```python
from build123d import *

# Parameters (mm, degrees)
EXTRUDE_1_DEPTH           = 12.5
CUT_EXTRUDE_1_DEPTH       = 20.532024985
CUT_EXTRUDE_1_DEPTH_BACK  = 20.532024985
SKETCH_2_R                = 2
CUT_EXTRUDE_2_DEPTH       = 20.532024985
CUT_EXTRUDE_2_DEPTH_BACK  = 20.532024985
CUT_EXTRUDE_START         = 12.5
SKETCH_5_W                = 16
SKETCH_5_H                = 5
CUT_EXTRUDE_4_DEPTH       = 5.5
CUT_EXTRUDE_5_DEPTH       = 2.5
CUT_EXTRUDE_5_DEPTH_BACK  = 2.5
EXTRUDE_START             = 12.5
EXTRUDE_5_DEPTH           = 1.5
SKETCH_8_R                = 1
CUT_EXTRUDE_6_DEPTH       = 1.5
CUT_EXTRUDE_START_2       = 14
CUT_EXTRUDE_7_DEPTH       = 1.5
CUT_EXTRUDE_9_DEPTH       = 29.943911277
CUT_EXTRUDE_9_DEPTH_BACK  = 29.943911277
CUT_EXTRUDE_10_DEPTH      = 29.943911277
CUT_EXTRUDE_10_DEPTH_BACK = 29.943911277


with BuildPart() as part:
    # 草图1 → 凸台-拉伸1 (new body)
    with BuildSketch(Plane(origin=(0, 0, 0), x_dir=(1, 0, 0), z_dir=(0, 1, 0))):
        Polygon((13, 5.5), (8, 5.5), (8, -5.5), (13, -5.5), (13, -7.5), (-13, -7.5), (-13, -5.5), (-8, -5.5), (-8, 5.5), (-13, 5.5), (-13, 7.5), (13, 7.5), align=None)
    extrude(amount=EXTRUDE_1_DEPTH)

    # 草图2 → 切除-拉伸1 (cut, two sides: drawn at the far end of the back side and taken through both)
    with BuildSketch(Plane.XY.offset(-CUT_EXTRUDE_1_DEPTH_BACK)):
        with Locations((0, 3.5)):
            Circle(SKETCH_2_R)
    extrude(amount=CUT_EXTRUDE_1_DEPTH + CUT_EXTRUDE_1_DEPTH_BACK, mode=Mode.SUBTRACT)

    # 草图3 → 切除-拉伸2 (cut, two sides: drawn at the far end of the back side and taken through both)
    with BuildSketch(Plane.XY.offset(-CUT_EXTRUDE_2_DEPTH_BACK)):
        with BuildLine():
            Line((-10.5, 11), (-2, 11))
            ThreePointArc((-2, 11), (-1, 10), (-2, 9))
            Line((-2, 9), (-10.5, 9))
            ThreePointArc((-10.5, 9), (-11.5, 10), (-10.5, 11))
        make_face()
        with BuildLine():
            Line((2, 9), (10.5, 9))
            ThreePointArc((10.5, 9), (11.5, 10), (10.5, 11))
            Line((10.5, 11), (2, 11))
            ThreePointArc((2, 11), (1, 10), (2, 9))
        make_face()
    extrude(amount=CUT_EXTRUDE_2_DEPTH + CUT_EXTRUDE_2_DEPTH_BACK, mode=Mode.SUBTRACT)

    # 草图5 → 切除-拉伸4 (cut)
    with BuildSketch(Plane(origin=(0, 0, 0), x_dir=(1, 0, 0), z_dir=(0, 1, 0)).offset(CUT_EXTRUDE_START)):
        Rectangle(SKETCH_5_W, SKETCH_5_H)
    extrude(amount=-CUT_EXTRUDE_4_DEPTH, mode=Mode.SUBTRACT)

    # 草图6 → 切除-拉伸5 (cut, two sides: drawn at the far end of the back side and taken through both)
    with BuildSketch(Plane.XY.offset(-CUT_EXTRUDE_5_DEPTH_BACK)):
        with BuildLine():
            Line((8, 7), (0, 7))
            ThreePointArc((0, 7), (4.949747468, 4.949747468), (7, 0))
            Line((7, 0), (8, 0))
            Line((8, 0), (8, 7))
        make_face()
        with BuildLine():
            Line((-8, 7), (-8, 0))
            Line((-8, 0), (-7, 0))
            ThreePointArc((-7, 0), (-4.949747468, 4.949747468), (0, 7))
            Line((0, 7), (-8, 7))
        make_face()
    extrude(amount=CUT_EXTRUDE_5_DEPTH + CUT_EXTRUDE_5_DEPTH_BACK, mode=Mode.SUBTRACT)

    # 草图7 → 凸台-拉伸5 (add)
    with BuildSketch(Plane(origin=(0, 0, 0), x_dir=(1, 0, 0), z_dir=(0, 1, 0)).offset(EXTRUDE_START)):
        with BuildLine():
            Line((17.82554347, 2.5), (15.07554347, 2.5))
            Line((15.07554347, 2.5), (15.07554347, -2.5))
            Line((15.07554347, -2.5), (17.82554347, -2.5))
            ThreePointArc((17.82554347, -2.5), (0, -18), (-17.82554347, -2.5))
            Line((-17.82554347, -2.5), (-15.07554347, -2.5))
            Line((-15.07554347, -2.5), (-15.07554347, 2.5))
            Line((-15.07554347, 2.5), (-17.82554347, 2.5))
            ThreePointArc((-17.82554347, 2.5), (0, 18), (17.82554347, 2.5))
        make_face()
    extrude(amount=EXTRUDE_5_DEPTH)

    # 草图8 → 切除-拉伸6 (cut)
    with BuildSketch(Plane(origin=(0, 0, 0), x_dir=(1, 0, 0), z_dir=(0, 1, 0)).offset(CUT_EXTRUDE_START)):
        with Locations(Location((0, 12.5, 0), (0, 0, 270))):
            Circle(SKETCH_8_R)
        with Locations(Location((0, -12.5, 0), (0, 0, 270))):
            Circle(SKETCH_8_R)
    extrude(amount=CUT_EXTRUDE_6_DEPTH, mode=Mode.SUBTRACT)

    # 草图9 → 切除-拉伸7 (cut)
    with BuildSketch(Plane(origin=(0, 0, 0), x_dir=(1, 0, 0), z_dir=(0, 1, 0)).offset(CUT_EXTRUDE_START_2)):
        with BuildLine():
            Line((-12.02081528, 10.606601718), (-13.435028843, 12.02081528))
            ThreePointArc((-13.435028843, 12.02081528), (-13.435028843, 13.435028843), (-12.02081528, 13.435028843))
            Line((-12.02081528, 13.435028843), (-10.606601718, 12.02081528))
            ThreePointArc((-10.606601718, 12.02081528), (-10.606601718, 10.606601718), (-12.02081528, 10.606601718))
        make_face()
        with BuildLine():
            Line((10.606601718, -12.02081528), (12.02081528, -13.435028843))
            ThreePointArc((12.02081528, -13.435028843), (13.435028843, -13.435028843), (13.435028843, -12.02081528))
            Line((13.435028843, -12.02081528), (12.02081528, -10.606601718))
            ThreePointArc((12.02081528, -10.606601718), (10.606601718, -10.606601718), (10.606601718, -12.02081528))
        make_face()
        with BuildLine():
            Line((-12.02081528, -10.606601718), (-13.435028843, -12.02081528))
            ThreePointArc((-13.435028843, -12.02081528), (-13.435028843, -13.435028843), (-12.02081528, -13.435028843))
            Line((-12.02081528, -13.435028843), (-10.606601718, -12.02081528))
            ThreePointArc((-10.606601718, -12.02081528), (-10.606601718, -10.606601718), (-12.02081528, -10.606601718))
        make_face()
        with BuildLine():
            Line((10.606601718, 12.02081528), (12.02081528, 13.435028843))
            ThreePointArc((12.02081528, 13.435028843), (13.435028843, 13.435028843), (13.435028843, 12.02081528))
            Line((13.435028843, 12.02081528), (12.02081528, 10.606601718))
            ThreePointArc((12.02081528, 10.606601718), (10.606601718, 10.606601718), (10.606601718, 12.02081528))
        make_face()
    extrude(amount=-CUT_EXTRUDE_7_DEPTH, mode=Mode.SUBTRACT)

    # 草图10 → 切除-拉伸9 (cut, two sides: drawn at the far end of the back side and taken through both)
    with BuildSketch(Plane.XY.offset(-CUT_EXTRUDE_9_DEPTH_BACK)):
        with BuildLine():
            Line((-11.5, 10), (-11.5, 3))
            ThreePointArc((-11.5, 3), (-10.5, 2), (-9.5, 3))
            Line((-9.5, 3), (-9.5, 10))
            ThreePointArc((-9.5, 10), (-10.5, 11), (-11.5, 10))
        make_face()
        with BuildLine():
            Line((11.5, 10), (11.5, 3))
            ThreePointArc((11.5, 3), (10.5, 2), (9.5, 3))
            Line((9.5, 3), (9.5, 10))
            ThreePointArc((9.5, 10), (10.5, 11), (11.5, 10))
        make_face()
    extrude(amount=CUT_EXTRUDE_9_DEPTH + CUT_EXTRUDE_9_DEPTH_BACK, mode=Mode.SUBTRACT)

    # 草图11 → 切除-拉伸10 (cut, two sides: drawn at the far end of the back side and taken through both)
    with BuildSketch(Plane.XY.offset(-CUT_EXTRUDE_10_DEPTH_BACK)):
        with BuildLine():
            Line((8.5, 9), (9.5, 9))
            Line((9.5, 9), (9.5, 8))
            ThreePointArc((9.5, 8), (9.207106781, 8.707106781), (8.5, 9))
        make_face()
        with BuildLine():
            Line((-9.5, 9), (-9.5, 8))
            ThreePointArc((-9.5, 8), (-9.207106781, 8.707106781), (-8.5, 9))
            Line((-8.5, 9), (-9.5, 9))
        make_face()
    extrude(amount=CUT_EXTRUDE_10_DEPTH + CUT_EXTRUDE_10_DEPTH_BACK, mode=Mode.SUBTRACT)


solid = part.part
```
Verification items for the finished model (mm, model axes). A direction names the side the tool comes from. Coordinates: 2 decimals unless noted, no trailing zeros. Write each loop counter-clockwise with the first axis right and the second up, starting at its lowest first coordinate (ties: lowest second). Pieces come first, ordered by that corner, then holes. Notation, with made-up numbers: M 16,-37.5 L 72,-37.5 A6 cw 72,-27.5 Z; hole C -16,24 d2. An arc over 180 degrees is marked long. One line per item, written item: value.
Item 1: Access from +Z, -Z, +X, -X, +Y, -Y to the whole of each face (thin tool, end or side, straight path). Record for faces 5 (the cylindrical face through (-16.295, 13.24, 7.646)), 6 (the cylindrical face through (-9.215, 8.699, 6.486)), 7 (the flat face through (8, 4, -4)), 8 (the flat face through (-8, 4, -4)), 9 (the flat face through (0, 6, 7.5)).
Check sheet entries:
face 5: +Z, -X, +Y, -Y
face 6: +Z, -Z
face 7: +X, -Y
face 8: -X, -Y
face 9: +Z, +X, -X, -Y
Item 2: Section check A-A, the plane y = 11.5. Record the boundary of the cut face in (x, z).
Check sheet entries:
outline: M -13,-7.5 L 13,-7.5 L 13,-5.5 L 8,-5.5 L 8,-2.5 L -8,-2.5 L -8,-5.5 L -13,-5.5 Z; M -13,5.5 L -8,5.5 L -8,2.5 L 8,2.5 L 8,5.5 L 13,5.5 L 13,7.5 L -13,7.5 Z
Item 3: Section check C-C, the plane x = 6.5. Record the boundary of the cut face in (y, z).
Check sheet entries:
outline: M 0,-7.5 L 9,-7.5 L 9,-2.5 L 2.6,-2.5 L 2.6,2.5 L 9,2.5 L 9,7.5 L 0,7.5 Z; M 11,-7.5 L 12.5,-7.5 L 12.5,-16.79 L 14,-16.79 L 14,16.79 L 12.5,16.79 L 12.5,7.5 L 11,7.5 L 11,2.5 L 12.5,2.5 L 12.5,-2.5 L 11,-2.5 Z
Item 4: Scan lines: line 1 along Y through (x, z) = (0, -1.25); line 2 along Z through (x, y) = (-3.5, 8.75); line 3 along X through (y, z) = (3.5, -3.5). Record each from-to range of solid material in increasing order.
Check sheet entries:
line 1: y = 0 to 1.5, 5.5 to 7, 12.5 to 14
line 2: z = -7.5 to -2.5, 2.5 to 7.5
line 3: x = -8 to -2, 2 to 8
Item 5: Gauge pin test, flat ends, axial feed: pin 1 Ø8 at (x, y) = (-8.5, 9.5) entering from +Z; pin 2 Ø5.5 at (x, y) = (11.5, 7) entering from -Z; pin 3 Ø1.2 at (y, z) = (13.5, -1) entering from +X. Record the tip position at first contact, or that the pin passes through.
Check sheet entries:
pin 1: stops at z = 17.02
pin 2: stops at z = -7.5
pin 3: stops at x = 15.08
Item 6: Section check D-D, the plane z = 5. Record the boundary of the cut face in (x, y), plus the area to 3 significant figures.
Check sheet entries:
outline: M -17.29,12.5 L -8,12.5 L -8,11 L -2,11 A1 cw -2,9 L -8,9 L -8,0 L 8,0 L 8,9 L 2,9 A1 cw 2,11 L 8,11 L 8,12.5 L 17.29,12.5 L 17.29,14 L -17.29,14 Z; hole C 0,3.5 d4
area: 212 mm^2
Item 7: Mould release check, pull along X, two halves, no side actions. Record for faces 1 (the flat face through (-9.5, 5, -7)), 2 (the flat face through (-9.5, 5, 6)), 3 (the flat face through (12, 6, -5.5)), 4 (the flat face through (-8, 12, 4)): pulls with the +X half, pulls with the -X half, needs draft (parallel to the pull), parting line crosses it, or undercut.
Check sheet entries:
face 1: undercut
face 2: undercut
face 3: needs draft
face 4: pulls with the -X half
Item 8: Section check B-B, the plane z = 12.5. Record the boundary of the cut face in (x, y).
Check sheet entries:
outline: M -11.09,12.5 L -1,12.5 L -1,14 L -11.09,14 Z; M 1,12.5 L 11.09,12.5 L 11.09,14 L 1,14 Z
